Autodesk Inventor part; units mm, degrees
ref_plane "YZ Plane" through (0, 0, 0) normal (1, 0, 0) x (0, 1, 0)
ref_plane "XZ Plane" through (0, 0, 0) normal (0, 1, 0) x (-1, 0, 0)
ref_plane "XY Plane" through (0, 0, 0) normal (0, 0, 1) x (1, 0, 0)
sketch "Sketch1" plane through (0, 0, 0) normal (0, 1, 0) x (-1, 0, 0)
  circle A0 centre (0, 0) radius 9.75
  circle A1 centre (0, 0) radius 10.75
  dimension "d0" = 19.5
  dimension "d1" = 21.5
extrude "Extrusion1" add sketch "Sketch1" along normal blind 2 contours A0 | A1
sketch "Sketch2" plane through (0, 2, 0) normal (0, 1, 0) x (1, 0, 0)
  circle A0 centre (0, 0) radius 9.75
  dimension "d4" = 19.5
extrude "Extrusion2" cut sketch "Sketch2" against normal blind 1
sketch "Sketch3" plane through (0, 1, 0) normal (0, 1, 0) x (1, 0, 0)
  circle A0 centre (0, 0) radius 8.75
  dimension "d7" = 17.5
extrude "Extrusion3" cut sketch "Sketch3" against normal blind 1
sketch "Sketch4" plane through (0, 0, 0) normal (0, -1, 0) x (1, 0, 0)
  circle A0 centre (0, 0) radius 8.75
  circle A1 centre (0, 0) radius 9.75
  dimension "d10" = 19.5
extrude "Extrusion4" add sketch "Sketch4" along normal blind 6
properties part number "685ZZFlanged_Adapter_2mm"
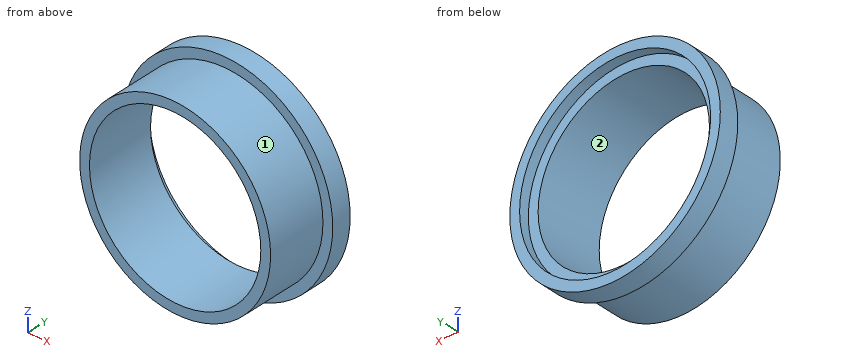
Geometry check sheet. Reference: the model listing, model coordinates, mm. Face numbers are marked on the shaded views. Round coordinates to 2 decimals unless told otherwise and drop trailing zeros. Loops run counter-clockwise (first coordinate to the right, second up) from the corner with the lowest first, then second, coordinate; pieces in that order, holes last. Notation, with made-up numbers: (-33, 68) -> (3, 68) arc R20 ccw to (3, 97) -> close; hole circle Ø8 at (-1, 0.25). An arc over 180 degrees is marked (long way). Answer as a JSON object with one key per item and string values. Group by question number.
Item 1: Depth check by flat-ended pin: pin 1 Ø2 at (x, y) = (1.5, -4) entering from +Z; pin 2 Ø8 at (x, z) = (8, -1) entering from +Y; pin 3 Ø6 at (x, z) = (-4, 4.5) entering from +Y; pin 4 Ø2 at (x, y) = (-1.5, -4.5) entering from -Z. Enter the tip coordinate at first touch or a pass-through.
Item 2: Cross-section at C-C, the plane y = -2. Record the cut outline in (x, z).
Item 3: Cross-section at A-A, the plane z = 0. Record the cut outline in (x, y).
Item 4: Cross-section at B-B, the plane x = 0. Record the cut outline in (y, z).
Item 5: Thickness scan on line 1 along Z through (x, y) = (0, 1.5); line 2 along Z through (x, y) = (0, -1.75); line 3 along X through (y, z) = (1.25, 7.5). Record the ranges inside material, lowest first.
Item 6: Release check for a two-part mould opening along X. For the marked faces 1 and 2 record: pulls with the +X half, pulls with the -X half, needs draft (parallel to the pull), parting line crosses it, or undercut.
Determined:
{
 "1": {"pin 1": "stops at z = 9.74", "pin 2": "stops at y = 2", "pin 3": "stops at y = 1", "pin 4": "stops at z = -9.74"},
 "2": {"outline": "circle Ø19.5 at (0, 0); hole circle Ø17.5 at (0, 0)"},
 "3": {"outline": "(-10.75, 0) -> (-9.75, 0) -> (-9.75, -6) -> (-8.75, -6) -> (-8.75, 1) -> (-9.75, 1) -> (-9.75, 2) -> (-10.75, 2) -> close; (8.75, -6) -> (9.75, -6) -> (9.75, 0) -> (10.75, 0) -> (10.75, 2) -> (9.75, 2) -> (9.75, 1) -> (8.75, 1) -> close"},
 "4": {"outline": "(-6, -9.75) -> (0, -9.75) -> (0, -10.75) -> (2, -10.75) -> (2, -9.75) -> (1, -9.75) -> (1, -8.75) -> (-6, -8.75) -> close; (-6, 8.75) -> (1, 8.75) -> (1, 9.75) -> (2, 9.75) -> (2, 10.75) -> (0, 10.75) -> (0, 9.75) -> (-6, 9.75) -> close"},
 "5": {"line 1": "z = -10.75 to -9.75, 9.75 to 10.75", "line 2": "z = -9.75 to -8.75, 8.75 to 9.75", "line 3": "x = -7.7 to -6.23, 6.23 to 7.7"},
 "6": {"face 1": "parting line crosses it", "face 2": "undercut"}
}
